Autodesk Inventor part; units mm, degrees
ref_plane "YZ Plane" through (0, 0, 0) normal (1, 0, 0) x (0, 1, 0)
ref_plane "XZ Plane" through (0, 0, 0) normal (0, 1, 0) x (-1, 0, 0)
ref_plane "XY Plane" through (0, 0, 0) normal (0, 0, 1) x (1, 0, 0)
sketch "Sketch1" plane through (0, 0, 0) normal (0, 0, 1) x (1, 0, 0)
  line L0 (-19, 24.7) -> (9.5, 24.7)
  line L1 (9.5, 24.7) -> (9.5, -21.8)
  line L2 (9.5, -21.8) -> (-19, -21.8)
  line L3 (-19, -21.8) -> (-19, 24.7)
  line L4 (-19, 21.4) -> (9.5, 21.4) construction
  line L5 (-4.75, 24.7) -> (-4.75, -21.8) construction
  circle A0 centre (-4.75, 13.27) radius 9.525
  circle A1 centre (-15.7, 21.4) radius 1.5
  line L6 (9.5, 1.45) -> (-19, 1.45) construction
  circle A2 centre (6.2, 21.4) radius 1.5
  circle A3 centre (-15.7, -18.5) radius 1.5
  circle A4 centre (6.2, -18.5) radius 1.5
  circle A5 centre (-4.75, 13.27) radius 2.5
  circle A6 centre (-4.75, 13.27) radius 4.2333
  line L7 (-4.75, 13.27) -> (-4.75, 22.795) construction
  circle A7 centre (-4.75, 21.4) radius 0.75
  circle A8 centre (-10.4988, 19.0188) radius 0.75
  circle A9 centre (-12.88, 13.27) radius 0.75
  circle A10 centre (-10.4988, 7.5212) radius 0.75
  circle A11 centre (-4.75, 5.14) radius 0.75
  circle A12 centre (0.9988, 7.5212) radius 0.75
  circle A13 centre (3.38, 13.27) radius 0.75
  circle A14 centre (0.9988, 19.0188) radius 0.75
  point P0 (0, 0)
  dimension "d2" = 19.05
  dimension "d0" = 28.5
  dimension "d1" = 46.5
  dimension "d3" = 11.43
  dimension "d4" = 3.3
  dimension "d5" = 3.3
  dimension "d6" = 3
  dimension "d7" = 5
  dimension "d8" = 8.4667
  dimension "d11" = 360
  dimension "d13" = 1.5
extrude "Extrusion1" add sketch "Sketch1" against normal blind 34 contours L0 L1 L2 L3 | A0 | A5 | A6 | A7 | A8 | A9 | A10 | A11 | A12 | A13 | A14
chamfer "Chamfer1" distance 2 angle 45 4 edges at (9.5, 24.7, -17) (-19, 24.7, -17) (9.5, -21.8, -17) (-19, -21.8, -17)
extrude "Extrusion2" add sketch "Sketch1" along normal blind 2 contours A0 | A6
extrude "Extrusion3" add sketch "Sketch1" along normal blind 2.5 contours A6
sketch "Sketch2" plane through (-19, -19.8, 0) normal (-1, 0, 0) x (0, 0, 1)
  line L0 (0, 42.5) -> (0, 0)
  line L1 (0, 10.7) -> (-34, 10.7)
  line L2 (-34, 0) -> (-34, 42.5)
  line L3 (-34, -2) -> (0, -2)
  circle A0 centre (-9.253, 10.7) radius 1.27
  circle A1 centre (-24.747, 10.7) radius 1.27
  point P0 (0, 19.8)
  dimension "d23" = 12.7
  dimension "d24" = 2.54
  dimension "d25" = 2.54
  dimension "d26" = 15.494
  dimension "d27" = 9.253
  dimension "d28" = 9.253
hole "Hole1" at (-19, -9.1, -9.253) at (-19, -9.1, -24.747) direction (1, 0, 0) diameter 2.54 end through all
equation "\"d28\" = d27"
properties part number "UpperArmServoDynamixelXM430-W350-T"
Here's how the part is built. I have some questions about the finished solid (model axes, mm). A direction names the side the tool comes from. Coordinates: 2 decimals unless noted, no trailing zeros. Order: outer loops, then holes, each group sorted by start corner. A loop starts at its lowest first (then second) coordinate and runs counter-clockwise, first axis right, second up.
Item 1: For P1, Ø0.8, axis at x = -10.5, y = 19, coming from the +Z side; P2, Ø4, axis at y = -9.1, z = -24.747, coming from the +X side; P3, Ø2, axis at x = -10.5, y = 19.02, coming from the +Z side, each with a flat end and sliding along its axis, tell me the tip position at first contact or that it passes through.
Result sheet:
P1: stops at z = 0
P2: stops at x = 9.5
P3: stops at z = 2
Item 2: For faces 4 (the face through (1, 8, 0)), 5 (the face through (6.005, -17.013, -16.762)), which set-ups out of +Z, -Z, +X, -X, +Y, -Y let a thin tool reach every point of the face, with its end or its side?
Result sheet:
face 4: +Z
face 5: +Z, -Z
Item 3: If we mould it in two halves opening along Y, with no side actions, what happens to faces 1 (the face through (-3, 11, 2.5)), 2 (the face through (1, 19, 0)), 3 (the face through (-12.309, 19.066, 0.986))? For each: +Y half, -Y half, draft (parallel to the pull), parting line (faces both ways), or undercut.
Result sheet:
face 1: draft
face 2: undercut
face 3: parting line
Item 4: I need wall thicknesses on line 1 (Y direction, x = 6.2, z = -26.5); line 2 (X direction, y = 21, z = -11); line 3 (Z direction, x = -13, y = -11). Which ranges of each line are inside material? Lowest first, please.
Result sheet:
line 1: y = -21.8 to -20, -17 to 19.9, 22.9 to 24.7
line 2: x = -19 to -17.15, -14.25 to 4.75, 7.65 to 9.5
line 3: z = -34 to 0
Item 5: If we section it at A-A on x = -15.7: List the corners of the cut face in (y, z) for me.
Result sheet:
outline: (-21.8, -34) - (-20, -34) - (-20, 0) - (-21.8, 0) - close; (-17, -34) - (19.9, -34) - (19.9, 0) - (-17, 0) - close; (22.9, -34) - (24.7, -34) - (24.7, 0) - (22.9, 0) - close; hole circle Ø2.54 at (-9.1, -24.75); hole circle Ø2.54 at (-9.1, -9.25)
Item 6: If we section it at C-C on z = -16.5: List the corners of the cut face in (x, y) for me.
Result sheet:
outline: (-19, -19.8) - (-17, -21.8) - (7.5, -21.8) - (9.5, -19.8) - (9.5, 22.7) - (7.5, 24.7) - (-17, 24.7) - (-19, 22.7) - close; hole circle Ø3 at (-15.7, -18.5); hole circle Ø3 at (-15.7, 21.4); hole circle Ø3 at (6.2, -18.5); hole circle Ø3 at (6.2, 21.4)
Item 7: If we section it at B-B on y = -9.1: List the corners of the cut face in (x, z) for me, plus the area to 3 significant figures.
Result sheet:
outline: (-19, -34) - (9.5, -34) - (9.5, -26.02) - (-19, -26.02) - close; (-19, -23.48) - (9.5, -23.48) - (9.5, -10.52) - (-19, -10.52) - close; (-19, -7.98) - (9.5, -7.98) - (9.5, 0) - (-19, 0) - close
area: 824 mm2
Item 8: If we section it at D-D on x = -4.75: List the corners of the cut face in (y, z) for me (3 decimals).
Result sheet:
outline: (-21.8, -34) - (24.7, -34) - (24.7, 0) - (22.795, 0) - (22.795, 2) - (22.15, 2) - (22.15, 0) - (20.65, 0) - (20.65, 2) - (17.503, 2) - (17.503, 2.5) - (15.77, 2.5) - (15.77, 0) - (10.77, 0) - (10.77, 2.5) - (9.037, 2.5) - (9.037, 2) - (5.89, 2) - (5.89, 0) - (4.39, 0) - (4.39, 2) - (3.745, 2) - (3.745, 0) - (-21.8, 0) - close; hole circle Ø2.54 at (-9.1, -24.747); hole circle Ø2.54 at (-9.1, -9.253)
